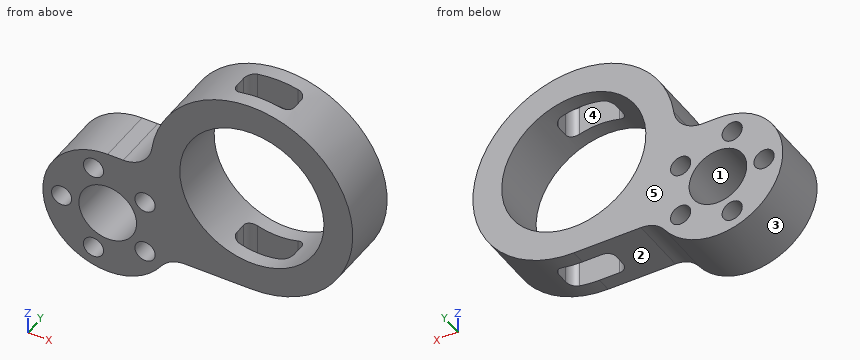
```python
from build123d import *

# Parameters (mm, degrees)
SKETCH1_R               = 12.5
SKETCH1_R_2             = 5
SKETCH1_R_3             = 1.75
BOSS_EXTRUDE1_DEPTH     = 10
CUT_EXTRUDE1_DEPTH      = 45.869499914
CUT_EXTRUDE1_DEPTH_BACK = 45.869499914


with BuildPart() as part:
    # Sketch1 → Boss-Extrude1 (new body)
    with BuildSketch(Plane(origin=(0, 0, 0), x_dir=(1, 0, 0), z_dir=(0, 1, 0))):
        with BuildLine():
            Line((-25, 1.978756555), (-22.29623484, 1.978756555))
            ThreePointArc((-22.29623484, 1.978756555), (-19.006625225, 0.744187285), (-17.341515987, -2.349856013))
            ThreePointArc((-17.341515987, -2.349856013), (13.179007554, -11.513633653), (0, 17.5))
            Line((0, 17.5), (-11.654343591, 17.5))
            ThreePointArc((-11.654343591, 17.5), (-13.971297253, 18.069229669), (-15.760699409, 19.647309709))
            ThreePointArc((-15.760699409, 19.647309709), (-34.969233245, 18.441902296), (-25, 1.978756555))
        make_face()
        with Locations(Location((0, 0, 0), (0, 0, 270))):
            Circle(SKETCH1_R, mode=Mode.SUBTRACT)
        with Locations(Location((-25, 13.228756555, 0), (0, 0, 270))):
            Circle(SKETCH1_R_2, mode=Mode.SUBTRACT)
        with Locations(Location((-33, 13.228756555, 0), (0, 0, 270))):
            Circle(SKETCH1_R_3, mode=Mode.SUBTRACT)
        with Locations(Location((-27.472135955, 20.837208686, 0), (0, 0, 270))):
            Circle(SKETCH1_R_3, mode=Mode.SUBTRACT)
        with Locations(Location((-18.527864045, 17.931038574, 0), (0, 0, 270))):
            Circle(SKETCH1_R_3, mode=Mode.SUBTRACT)
        with Locations(Location((-18.527864045, 8.526474537, 0), (0, 0, 270))):
            Circle(SKETCH1_R_3, mode=Mode.SUBTRACT)
        with Locations(Location((-27.472135955, 5.620304425, 0), (0, 0, 270))):
            Circle(SKETCH1_R_3, mode=Mode.SUBTRACT)
    extrude(amount=BOSS_EXTRUDE1_DEPTH)

    # Sketch2 → Cut-Extrude1 (cut, two sides: drawn at the far end of the back side and taken through both)
    with BuildSketch(Plane.XY.offset(-CUT_EXTRUDE1_DEPTH_BACK)):
        with BuildLine():
            Line((-3.5, 7.5), (3.5, 7.5))
            ThreePointArc((3.5, 7.5), (4.560660172, 7.060660172), (5, 6))
            Line((5, 6), (5, 4))
            ThreePointArc((5, 4), (4.560660172, 2.939339828), (3.5, 2.5))
            Line((3.5, 2.5), (-3.5, 2.5))
            ThreePointArc((-3.5, 2.5), (-4.560660172, 2.939339828), (-5, 4))
            Line((-5, 4), (-5, 6))
            ThreePointArc((-5, 6), (-4.560660172, 7.060660172), (-3.5, 7.5))
        make_face()
    extrude(amount=CUT_EXTRUDE1_DEPTH + CUT_EXTRUDE1_DEPTH_BACK, mode=Mode.SUBTRACT)


solid = part.part
```
Build history of the part. All positions in model axes, mm. Face numbers are marked on the shaded views. A direction names the side the tool comes from. Round coordinates to 2 decimals unless told otherwise and drop trailing zeros. Write each loop counter-clockwise with the first axis right and the second up, starting at its lowest first coordinate (ties: lowest second). Pieces come first, ordered by that corner, then holes.
1) Drill centre lines: probe 1 along X at (y, z) = (4, -7.5); probe 2 along Z at (x, y) = (-18, 2); probe 3 along X at (y, z) = (7.25, -12). Where is each one in solid material? Low to high.
2) Mould opens along X. For the marked faces 1, 2 and 3 say: +X half, -X half, draft (parallel to the pull), parting line (faces both ways), or undercut.
3) Band-saw the part on B-B, the plane x = -1. List the corners of the cut face in (y, z), and give its area (3 significant figures).
4) 3-axis set-ups, long thin cutter, end or side, ignore diameter. For the marked faces 4 and 5: which of +Z, -Z, +X, -X, +Y, -Y reach the whole face in a straight line?
5) Band-saw the part on A-A, the plane y = 5.25. List the corners of the cut face in (x, z).
6) Pin check, flat tips, straight feed: pin 1 (3 mm diameter, centred on y = 8.5, z = 4.5, fed in from -X); pin 2 (0.8 mm diameter, centred on x = -24.5, y = 4, fed in from +Z); pin 3 (1.6 mm diameter, centred on y = 4.5, z = 13.5, fed in from +X). Stop position of each tip, or through.
7) Band-saw the part on C-C, the plane z = 9. List the corners of the cut face in (x, y), and give its area (3 significant figures).
8) Band-saw the part on D-D, the plane x = -33. List the corners of the cut face in (y, z), and give its area (3 significant figures).
Ans:
1. probe 1: x = -34.68 to -19.95, -17.11 to -10, 10 to 15.81
1. probe 2: z = -22.04 to -19.6, -16.26 to -10.19, -6.86 to 0.46
1. probe 3: x = -36.18 to -34.25, -31.75 to -29.85, -20.15 to -4.33, 4.33 to 12.74
2. face 1: undercut
2. face 2: draft
2. face 3: parting line
3. outline: (0, -17.5) - (2.5, -17.5) - (2.5, -12.46) - (0, -12.46) - close; (0, 12.46) - (2.5, 12.46) - (2.5, 17.47) - (0, 17.47) - close; (7.5, -17.5) - (10, -17.5) - (10, -12.46) - (7.5, -12.46) - close; (7.5, 12.46) - (10, 12.46) - (10, 17.47) - (7.5, 17.47) - close
3. area: 50.3 mm2
4. face 4: +Z, -Z
4. face 5: +Z, -Z, +X, -X, +Y
5. outline: (-25, -1.98) arc R11.25 ccw (long way) to (-15.76, -19.65) arc R5 cw to (-11.65, -17.5) - (-5, -17.5) - (-5, -11.46) arc R12.5 cw to (-5, 11.46) - (-5, 16.77) arc R17.5 ccw to (-17.34, 2.35) arc R5 cw to (-22.3, -1.98) - close; (5, -16.77) arc R17.5 ccw to (5, 16.77) - (5, 11.46) arc R12.5 cw to (5, -11.46) - close; hole circle Ø3.5 at (-33, -13.23); hole circle Ø10 at (-25, -13.23); hole circle Ø3.5 at (-27.47, -20.84); hole circle Ø3.5 at (-27.47, -5.62); hole circle Ø3.5 at (-18.53, -17.93); hole circle Ø3.5 at (-18.53, -8.53)
6. pin 1: stops at x = -17.24
6. pin 2: stops at z = -1.98
6. pin 3: stops at x = 12.04
7. outline: (-15.01, 0) - (-8.67, 0) - (-8.67, 10) - (-15.01, 10) - close; (8.67, 0) - (15.01, 0) - (15.01, 10) - (8.67, 10) - close
7. area: 127 mm2
8. outline: (0, -21.14) - (10, -21.14) - (10, -14.98) - (0, -14.98) - close; (0, -11.48) - (10, -11.48) - (10, -5.32) - (0, -5.32) - close
8. area: 123 mm2
